Geometry: final body of the model. Coordinates: model frame, mm. A direction names the side the tool comes from. Give positions to 0.01 mm unless a question says otherwise; leave off trailing zeros. Write each loop counter-clockwise with the first axis right and the second up, starting at its lowest first coordinate (ties: lowest second). Pieces come first, ordered by that corner, then holes. Notation, with made-up numbers: (62.25, 32.25) - (77.25, 32.25) arc R18 ccw to (77.25, 64.25) - close; hole circle Ø10 at (5.5, 48). An arc over 180 degrees is marked (long way). Use CSV: the item, a comma, the result in double quotes. Start each with the question number.
(1) Section C-C on z = 0.9. Output: boundary loops of the cut face in (x, y).
(2) Section A-A on x = -8. Output: boundary loops of the cut face in (y, z).
(3) Reachability of faces 4 (the flat face through (-66, -32, 2)), 5 (the cylindrical face through (-15, -35.5, 1.5)) from +Z, -Z, +X, -X, +Y, -Y: full face, straight path, thin tool, end or side. Return the list, or none.
(4) Section D-D on x = -15. Output: boundary loops of the cut face in (y, z).
(5) Section B-B on y = -7. Output: boundary loops of the cut face in (x, z), and give its area (3 significant figures).
(6) Draft query along Y for faces 1 (the flat face through (-33, -26, 0)), 2 (the flat face through (-33, -65, 2)), 3 (the cylindrical face through (-8, -58, 1)). Return one class per face: released by +Y, released by -Y, zero draft, split by the parting line, or undercut.
(7) Line query: probe 1 along Y at (x, z) = (-58, 1.5); probe 2 along X at (y, z) = (-8, 2.15); probe 3 along X at (y, z) = (-43, 1.45). Output: solid intervals per line, ascending. Write a range as [from, to].
from build123d import *

# Parameters (mm, degrees)
SKETCH1_W           = 3
SKETCH1_H           = 65
BOSS_EXTRUDE1_DEPTH = 66
CUT_EXTRUDE3_REACH  = 5
SKETCH5_R           = 2


with BuildPart() as part:
    # Sketch1 → Boss-Extrude1 (new body)
    with BuildSketch(Plane(origin=(0, 0, 0), x_dir=(0, 0, -1), z_dir=(1, 0, 0))):
        with Locations((-1.5, -32.5)):
            Rectangle(SKETCH1_W, SKETCH1_H)
    extrude(amount=-BOSS_EXTRUDE1_DEPTH)

    # Sketch5 → Cut-Extrude3 (cut, up to next)
    with BuildSketch(Plane(origin=(0, 0, 0), x_dir=(-1, 0, 0), z_dir=(0, 0, -1)), mode=Mode.PRIVATE) as cut_extrude3_sk1:
        with Locations((8, -7)):
            Circle(SKETCH5_R)
    cut_extrude3_tool1 = extrude(cut_extrude3_sk1.sketch, amount=-CUT_EXTRUDE3_REACH, mode=Mode.PRIVATE) & part.part
    add(cut_extrude3_tool1.solids().sort_by_distance((-8, -7, 0))[0], mode=Mode.SUBTRACT)
    # Sketch5 → Cut-Extrude3 (cut, up to next)
    with BuildSketch(Plane(origin=(0, 0, 0), x_dir=(-1, 0, 0), z_dir=(0, 0, -1)), mode=Mode.PRIVATE) as cut_extrude3_sk2:
        with Locations((58, -7)):
            Circle(SKETCH5_R)
    cut_extrude3_tool2 = extrude(cut_extrude3_sk2.sketch, amount=-CUT_EXTRUDE3_REACH, mode=Mode.PRIVATE) & part.part
    add(cut_extrude3_tool2.solids().sort_by_distance((-58, -7, 0))[0], mode=Mode.SUBTRACT)
    # Sketch5 → Cut-Extrude3 (cut, up to next)
    with BuildSketch(Plane(origin=(0, 0, 0), x_dir=(-1, 0, 0), z_dir=(0, 0, -1)), mode=Mode.PRIVATE) as cut_extrude3_sk3:
        with Locations((8, -60)):
            Circle(SKETCH5_R)
    cut_extrude3_tool3 = extrude(cut_extrude3_sk3.sketch, amount=-CUT_EXTRUDE3_REACH, mode=Mode.PRIVATE) & part.part
    add(cut_extrude3_tool3.solids().sort_by_distance((-8, -60, 0))[0], mode=Mode.SUBTRACT)
    # Sketch5 → Cut-Extrude3 (cut, up to next)
    with BuildSketch(Plane(origin=(0, 0, 0), x_dir=(-1, 0, 0), z_dir=(0, 0, -1)), mode=Mode.PRIVATE) as cut_extrude3_sk4:
        with Locations((58, -60)):
            Circle(SKETCH5_R)
    cut_extrude3_tool4 = extrude(cut_extrude3_sk4.sketch, amount=-CUT_EXTRUDE3_REACH, mode=Mode.PRIVATE) & part.part
    add(cut_extrude3_tool4.solids().sort_by_distance((-58, -60, 0))[0], mode=Mode.SUBTRACT)
    # Sketch5 → Cut-Extrude3 (cut, up to next)
    with BuildSketch(Plane(origin=(0, 0, 0), x_dir=(-1, 0, 0), z_dir=(0, 0, -1)), mode=Mode.PRIVATE) as cut_extrude3_sk5:
        with BuildLine():
            Line((38, -37.5), (38, -42.5))
            ThreePointArc((38, -42.5), (33, -47.5), (28, -42.5))
            Line((28, -42.5), (28, -37.5))
            ThreePointArc((28, -37.5), (33, -32.5), (38, -37.5))
        make_face()
    cut_extrude3_tool5 = extrude(cut_extrude3_sk5.sketch, amount=-CUT_EXTRUDE3_REACH, mode=Mode.PRIVATE) & part.part
    add(cut_extrude3_tool5.solids().sort_by_distance((-33, -40, 0))[0], mode=Mode.SUBTRACT)
    # Sketch5 → Cut-Extrude3 (cut, up to next)
    with BuildSketch(Plane(origin=(0, 0, 0), x_dir=(-1, 0, 0), z_dir=(0, 0, -1)), mode=Mode.PRIVATE) as cut_extrude3_sk6:
        with BuildLine():
            Line((17, -37.5), (17, -42.5))
            ThreePointArc((17, -42.5), (15, -44.5), (13, -42.5))
            Line((13, -42.5), (13, -37.5))
            ThreePointArc((13, -37.5), (15, -35.5), (17, -37.5))
        make_face()
    cut_extrude3_tool6 = extrude(cut_extrude3_sk6.sketch, amount=-CUT_EXTRUDE3_REACH, mode=Mode.PRIVATE) & part.part
    add(cut_extrude3_tool6.solids().sort_by_distance((-15, -40, 0))[0], mode=Mode.SUBTRACT)
    # Sketch5 → Cut-Extrude3 (cut, up to next)
    with BuildSketch(Plane(origin=(0, 0, 0), x_dir=(-1, 0, 0), z_dir=(0, 0, -1)), mode=Mode.PRIVATE) as cut_extrude3_sk7:
        with BuildLine():
            Line((53, -37.5), (53, -42.5))
            ThreePointArc((53, -42.5), (51, -44.5), (49, -42.5))
            Line((49, -42.5), (49, -37.5))
            ThreePointArc((49, -37.5), (51, -35.5), (53, -37.5))
        make_face()
    cut_extrude3_tool7 = extrude(cut_extrude3_sk7.sketch, amount=-CUT_EXTRUDE3_REACH, mode=Mode.PRIVATE) & part.part
    add(cut_extrude3_tool7.solids().sort_by_distance((-51, -40, 0))[0], mode=Mode.SUBTRACT)


solid = part.part
Check values:
1,outline,"(-66, -65) - (0, -65) - (0, 0) - (-66, 0) - close; hole circle Ø4 at (-58, -60); hole circle Ø4 at (-58, -7); hole (-53, -42.5) arc R2 ccw to (-49, -42.5) - (-49, -37.5) arc R2 ccw to (-53, -37.5) - close; hole (-38, -42.5) arc R5 ccw to (-28, -42.5) - (-28, -37.5) arc R5 ccw to (-38, -37.5) - close; hole (-17, -42.5) arc R2 ccw to (-13, -42.5) - (-13, -37.5) arc R2 ccw to (-17, -37.5) - close; hole circle Ø4 at (-8, -60); hole circle Ø4 at (-8, -7)"
2,outline,"(-65, 0) - (-62, 0) - (-62, 3) - (-65, 3) - close; (-58, 0) - (-9, 0) - (-9, 3) - (-58, 3) - close; (-5, 0) - (0, 0) - (0, 3) - (-5, 3) - close"
3,face 4,"+Z, -Z, -X, +Y, -Y"
3,face 5,"+Z, -Z"
4,outline,"(-65, 0) - (-44.5, 0) - (-44.5, 3) - (-65, 3) - close; (-35.5, 0) - (0, 0) - (0, 3) - (-35.5, 3) - close"
5,outline,"(-66, 0) - (-60, 0) - (-60, 3) - (-66, 3) - close; (-56, 0) - (-10, 0) - (-10, 3) - (-56, 3) - close; (-6, 0) - (0, 0) - (0, 3) - (-6, 3) - close"
5,area,"174 mm²"
6,face 1,"zero draft"
6,face 2,"released by -Y"
6,face 3,"undercut"
7,probe 1,"y = [-65, -62], [-58, -9], [-5, 0]"
7,probe 2,"x = [-66, -59.73], [-56.27, -9.73], [-6.27, 0]"
7,probe 3,"x = [-66, -52.94], [-49.06, -37.97], [-28.03, -16.94], [-13.06, 0]"
